from build123d import *

# Parameters (mm, degrees)
SKETCH2_R           = 3
BOSS_EXTRUDE1_DEPTH = 30


with BuildPart() as part:
    # Sketch1 → Revolve1 (revolve)
    with BuildSketch(Plane.XY, mode=Mode.PRIVATE) as revolve1_sk:
        Polygon((0, 81.78), (0, 41.21), (8.33, 41.21), (10.015, 41.21), (10.015, 64.9), (8.45, 64.9), (8.45, 81.78), align=None)
    revolve(revolve1_sk.sketch.rotate(Axis((0, 0, 0), (0, 1, 0)), 90), axis=Axis((0, 0, 0), (0, 1, 0)))

    # Sketch1_3 → Revolve2 (revolve)
    with BuildSketch(Plane.XY, mode=Mode.PRIVATE) as revolve2_sk:
        Polygon((0, 41.21), (0, 0), (4.75, 0), (6, 29.21), (8.33, 35.21), (8.33, 41.21), align=None)
    revolve(revolve2_sk.sketch.rotate(Axis((0, 0, 0), (0, 1, 0)), 90), axis=Axis((0, 0, 0), (0, 1, 0)))

    # Sketch2 → Boss-Extrude1 (add)
    with BuildSketch(Plane.XZ):
        with Locations(Location((0, 0, 0), (0, 0, 270))):
            Circle(SKETCH2_R)
    extrude(amount=BOSS_EXTRUDE1_DEPTH)


solid = part.part
For this review, take the finished solid that the model builds, in its own axes (mm). A direction names the side the tool comes from. Give positions to 0.01 mm unless a question says otherwise; leave off trailing zeros. Order: outer loops, then holes, each group sorted by start corner. A loop starts at its lowest first (then second) coordinate and runs counter-clockwise, first axis right, second up. Notation, with made-up numbers: (52, -5) - (102, -5) arc R13 ccw to (102, 6) - close; hole circle Ø11 at (5, 21.25). An arc over 180 degrees is marked (long way). Answer as a JSON object with one key per item and string values. Group by question number.
Item 1: Take a section at B-B on x = 0. Give the boundary of the cut face in (y, z) (3 decimals).
Item 2: Take a section at C-C on y = -11. Give the boundary of the cut face in (x, z), and give its area (3 significant figures).
Item 3: Wall thickness on line 1 along Y through (x, z) = (2.75, -2.5); line 2 along Y through (x, z) = (7, -6.5); line 3 along X through (y, z) = (17.5, 0): over which ranges is each line inside the solid? List them lowest first.
Item 4: Machinability: for faces 1 (the flat face through (7, 64.9, 5)), 2 (the flat face through (0, 81.78, 0)), 3 (the cylindrical face through (7.39, 38.25, -3.84)), which of the approach directions +Z, -Z, +X, -X, +Y, -Y give a long, thin tool a straight path to every point of the face, cutting with its end or side? Answer none if there is none.
Item 5: Clearance check with flat-ended pins moving along their axes: pin 1 Ø1.5 at (y, z) = (-16, -3) entering from -X; pin 2 Ø12 at (x, y) = (3.5, 20.5) entering from -Z; pin 3 Ø10 at (x, z) = (7.5, 3) entering from -Y; pin 4 Ø8 at (y, z) = (-7, -7.5) entering from -X. State where each tip first meets the part, or that it passes through.
Item 6: Take a section at D-D on y = 21. Give the boundary of the cut face in (x, z).
Item 7: Take a section at A-A on z = 0. Give the boundary of the cut face in (x, y) (3 decimals), and give its area (3 significant figures).
Reported:
{
 "1": {"outline": "(-30, -3) - (0, -3) - (0, -4.75) - (29.21, -6) - (35.21, -8.33) - (41.21, -8.33) - (41.21, -10.015) - (64.9, -10.015) - (64.9, -8.45) - (81.78, -8.45) - (81.78, 8.45) - (64.9, 8.45) - (64.9, 10.015) - (41.21, 10.015) - (41.21, 8.33) - (35.21, 8.33) - (29.21, 6) - (0, 4.75) - (0, 3) - (-30, 3) - close"},
 "2": {"outline": "circle Ø6 at (0, 0)", "area": "28.3 mm^2"},
 "3": {"line 1": "0 to 81.78", "line 2": "41.21 to 64.9", "line 3": "-5.5 to 5.5"},
 "4": {"face 1": "+Y", "face 2": "+Z, -Z, +X, -X, +Y", "face 3": "-Y"},
 "5": {"pin 1": "x = -1.98", "pin 2": "z = -5.84", "pin 3": "y = 0", "pin 4": "through"},
 "6": {"outline": "circle Ø11.3 at (0, 0)"},
 "7": {"outline": "(-10.015, 41.21) - (-8.33, 41.21) - (-8.33, 35.21) - (-6, 29.21) - (-4.75, 0) - (-3, 0) - (-3, -30) - (3, -30) - (3, 0) - (4.75, 0) - (6, 29.21) - (8.33, 35.21) - (8.33, 41.21) - (10.015, 41.21) - (10.015, 64.9) - (8.45, 64.9) - (8.45, 81.78) - (-8.45, 81.78) - (-8.45, 64.9) - (-10.015, 64.9) - close", "area": "1,440 mm^2"}
}
